CAD build for the part. Positions are in the model's coordinates, mm. Face numbers are marked on the shaded views. A direction names the side the tool comes from. Round coordinates to 2 decimals unless told otherwise and drop trailing zeros. Write each loop counter-clockwise with the first axis right and the second up, starting at its lowest first coordinate (ties: lowest second). Pieces come first, ordered by that corner, then holes. Notation, with made-up numbers: (56, 12) -> (70, 12) arc R9 cw to (70, 18) -> close; hole circle Ø8 at (-22, -39). An arc over 180 degrees is marked (long way). Answer in a Markdown table with one row per item. Add a question column.
Autodesk Inventor part; units mm, degrees
ref_plane "YZ Plane" through (0, 0, 0) normal (1, 0, 0) x (0, 1, 0)
ref_plane "XZ Plane" through (0, 0, 0) normal (0, 1, 0) x (-1, 0, 0)
ref_plane "XY Plane" through (0, 0, 0) normal (0, 0, 1) x (1, 0, 0)
sketch "Sketch1" plane through (0, 0, 0) normal (0, 1, 0) x (-1, 0, 0)
  line L0 (-21, -21) -> (21, -21)
  line L1 (21, -21) -> (21, 21)
  line L2 (21, 21) -> (-21, 21)
  line L3 (-21, 21) -> (-21, -21)
  line L4 (-21, -21) -> (21, 21) construction
  line L5 (21, -21) -> (-21, 21) construction
  point P0 (0, 0)
  dimension "d0" = 42
  dimension "d1" = 42
extrude "Extrusion1" add sketch "Sketch1" along normal blind 8
sketch "Sketch2" plane through (0, 0, 0) normal (0, -1, 0) x (1, 0, 0)
  point P0 (0, 0)
chamfer "Chamfer1" distance 6 angle 45 4 edges at (-21, 4, 21) (21, 4, 21) (21, 4, -21) (-21, 4, -21)
sketch "Sketch3" plane through (0, 8, 0) normal (0, 1, 0) x (1, 0, 0)
  line L0 (-21, 15) -> (-15, 21)
  line L1 (-21, 15) -> (-21, -15)
  line L2 (-15, -21) -> (-21, -15)
  line L3 (-15, -21) -> (15, -21)
  line L4 (21, -15) -> (15, -21)
  line L5 (21, -15) -> (21, 15)
  line L6 (15, 21) -> (21, 15)
  line L7 (15, 21) -> (-15, 21)
  line L8 (-19.6609, -14.0495) -> (-13.6609, -20.0495)
  line L9 (-15, -21) -> (-21, -15)
  line L10 (-21, -15) -> (-19.8552, -13.8552)
  line L11 (-19.8552, -13.8552) -> (-19.6609, -14.0495)
  line L12 (-15, -21) -> (-13.8552, -19.8552)
  line L13 (-13.6609, -20.0495) -> (-13.1481, -20.5623)
  line L14 (-13.1481, -20.5623) -> (-13.5858, -21)
  line L15 (-19.8552, -13.8552) -> (-20.5623, -13.1481)
  line L16 (-20.5623, -13.1481) -> (-21, -13.5858)
  point P0 (0, 0)
  dimension "d11" = 1
  dimension "d12" = 1
extrude "Extrusion2" add sketch "Sketch3" along normal blind 2 contours L16 L15 L10 L1 | L10 L11 L8 L12 L2 | L12 L8 L13 L14 L3
mirror "Mirror1" about plane through (0, 0, 0) normal (0, 0, 1) of "Extrusion2"
mirror "Mirror2" about plane through (0, 0, 0) normal (1, 0, 0) of "Extrusion2", "Mirror1"
fillet "Fillet2" radius 1 8 edges at (15, 5, -21) (21, 5, -15) (21, 5, 15) (15, 5, 21) (-15, 5, 21) (-21, 5, 15) (-21, 5, -15) (-15, 5, -21)
fillet "Fillet3" radius 1 8 edges at (-21, 9, 13.5858) (-13.5858, 9, 21) (13.5858, 9, 21) (21, 9, 13.5858) (21, 9, -13.5858) (13.5858, 9, -21) (-13.5858, 9, -21) (-21, 9, -13.5858)
sketch "Sketch4" plane through (0, 0, 0) normal (0, -1, 0) x (1, 0, 0)
  circle A0 centre (0, 0) radius 16
  circle A1 centre (0, 0) radius 11
  dimension "d14" = 32
  dimension "d15" = 22
extrude "Extrusion3" cut sketch "Sketch4" against normal blind 1
sketch "Sketch5" plane through (0, 0, 0) normal (0, -1, 0) x (1, 0, 0)
  circle A0 centre (0, 0) radius 11
extrude "Extrusion4" add sketch "Sketch5" along normal blind 2.5
sketch "Sketch6" plane through (0, -2.5, 0) normal (0, -1, 0) x (1, 0, 0)
  circle A0 centre (0, 0) radius 4.5
  dimension "d20" = 9
extrude "Extrusion5" cut sketch "Sketch6" against normal up to surface (10.5 mm away)
sketch "Sketch7" plane through (0, 0, 0) normal (0, -1, 0) x (1, 0, 0)
  point P0 (0, 0)
sketch "Sketch8" plane through (0, 0, 0) normal (0, -1, 0) x (1, 0, 0)
  circle A0 centre (-15.5, -15.5) radius 1.5
  line L0 (14.5858, -21) -> (-14.5858, -21)
  line L1 (-21, -14.5858) -> (-21, 14.5858)
  point P0 (0, 0)
  dimension "d23" = 3
  dimension "d24" = 5.5
  dimension "d25" = 5.5
extrude "Extrusion6" cut sketch "Sketch8" against normal blind 5
mirror "Mirror3" about plane through (0, 0, 0) normal (0, 0, 1) of "Extrusion6"
mirror "Mirror4" about plane through (0, 0, 0) normal (1, 0, 0) of "Extrusion6", "Mirror3"
fillet "Fillet4" radius 0.5 1 edges at (-11, -2.5, 0)
fillet "Fillet5" radius 0.5 1 edges at (-4.5, -2.5, 0)
equation "\"d12\" = d11"
equation "\"d25\" = d24"
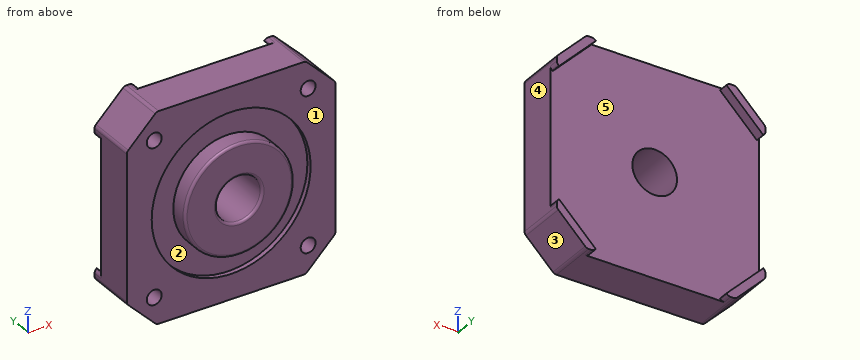
Item 1: Saw through at D-D on x = -16.5. Give the cut face in (y, z).
Item 2: Two-plate mould, pull along X, no slides. Class the marked faces 1, 2 and 3: +X half, -X half, draft (parallel to the pull), parting line (faces both ways), or undercut.
Item 3: Pin check, flat tips, straight feed: pin 1 (0.9 mm diameter, centred on x = -15, z = -16, fed in from -Y); pin 2 (10 mm diameter, centred on x = -15.5, z = -12, fed in from +Y); pin 3 (6 mm diameter, centred on x = -9.5, z = -1, fed in from +Y); pin 4 (7 mm diameter, centred on x = 0, z = 0, fed in from +Y) (3 decimals). Stop position of each tip, or through.
Item 4: Tool access for the marked faces 4 and 5: list every direction of +Z, -Z, +X, -X, +Y, -Y with a clear straight run to the whole face (end or side of a thin tool).
Item 5: Drill centre lines: probe 1 along Y at (x, z) = (-8, -2.5); probe 2 along Y at (x, z) = (-19, -6.5); probe 3 along Z at (x, y) = (-15.5, 2.2). Where is each one in solid material? Low to high.
Item 6: Saw through at C-C on y = 7.5. Give the cut face in (x, z), then the cut area to 3 significant figures.
Item 7: Saw through at A-A on y = 2.75. Give the cut face in (x, z), then the cut area to 3 significant figures.
Item 8: Saw through at B-B on x = 0. Give the cut face in (y, z), then the cut area to 3 significant figures.
Recorded:
| question | item | result |
|---|---|---|
| 1 | outline | (0, -19.5) -> (10, -19.5) -> (10, -17.21) -> (8, -17.21) -> (8, 17.21) -> (10, 17.21) -> (10, 19.5) -> (0, 19.5) -> (0, 16.62) -> (5, 16.62) -> (5, 14.38) -> (0, 14.38) -> (0, -14.38) -> (5, -14.38) -> (5, -16.62) -> (0, -16.62) -> close |
| 2 | face 1 | draft |
| 2 | face 2 | undercut |
| 2 | face 3 | +X half |
| 3 | pin 1 | y = 5 |
| 3 | pin 2 | y = 10 |
| 3 | pin 3 | y = 8 |
| 3 | pin 4 | through |
| 4 | face 4 | +Z, -Z, +X, +Y, -Y |
| 4 | face 5 | +Y |
| 5 | probe 1 | -2.5 to 8 |
| 5 | probe 2 | 0 to 8 |
| 5 | probe 3 | -20.5 to -17, -14 to 14, 17 to 20.5 |
| 6 | outline | (-21, -14.59) arc R1 ccw to (-20.71, -15.29) -> (-15.29, -20.71) arc R1 ccw to (-14.59, -21) -> (14.59, -21) arc R1 ccw to (15.29, -20.71) -> (20.71, -15.29) arc R1 ccw to (21, -14.59) -> (21, 14.59) arc R1 ccw to (20.71, 15.29) -> (15.29, 20.71) arc R1 ccw to (14.59, 21) -> (-14.59, 21) arc R1 ccw to (-15.29, 20.71) -> (-20.71, 15.29) arc R1 ccw to (-21, 14.59) -> close; hole circle Ø9 at (0, 0) |
| 6 | area | 1,630 mm2 |
| 7 | outline | (-21, -14.59) arc R1 ccw to (-20.71, -15.29) -> (-15.29, -20.71) arc R1 ccw to (-14.59, -21) -> (14.59, -21) arc R1 ccw to (15.29, -20.71) -> (20.71, -15.29) arc R1 ccw to (21, -14.59) -> (21, 14.59) arc R1 ccw to (20.71, 15.29) -> (15.29, 20.71) arc R1 ccw to (14.59, 21) -> (-14.59, 21) arc R1 ccw to (-15.29, 20.71) -> (-20.71, 15.29) arc R1 ccw to (-21, 14.59) -> close; hole circle Ø3 at (-15.5, -15.5); hole circle Ø3 at (-15.5, 15.5); hole circle Ø9 at (0, 0); hole circle Ø3 at (15.5, -15.5); hole circle Ø3 at (15.5, 15.5) |
| 7 | area | 1,600 mm2 |
| 8 | outline | (-2.5, -10.5) arc R0.5 ccw to (-2, -11) -> (1, -11) -> (1, -16) -> (0, -16) -> (0, -21) -> (8, -21) -> (8, -4.5) -> (-2, -4.5) arc R0.5 ccw to (-2.5, -5) -> close; (-2.5, 5) arc R0.5 ccw to (-2, 4.5) -> (8, 4.5) -> (8, 21) -> (0, 21) -> (0, 16) -> (1, 16) -> (1, 11) -> (-2, 11) arc R0.5 ccw to (-2.5, 10.5) -> close |
| 8 | area | 286 mm2 |
